Geometry check sheet. Reference: drawing and pictorial views, mm from the part's lowest x, y, z. A direction names the side the tool comes from. Coordinates: 2 decimals unless noted, no trailing zeros. Write each loop counter-clockwise with the first axis right and the second up, starting at its lowest first coordinate (ties: lowest second). Pieces come first, ordered by that corner, then holes. Notation, with made-up numbers: (34, 43.5) -> (45, 43.5) arc R23 ccw to (45, 67.5) -> close; hole circle Ø10 at (51.25, 38). An arc over 180 degrees is marked (long way). Answer in a Markdown table with one row per item.
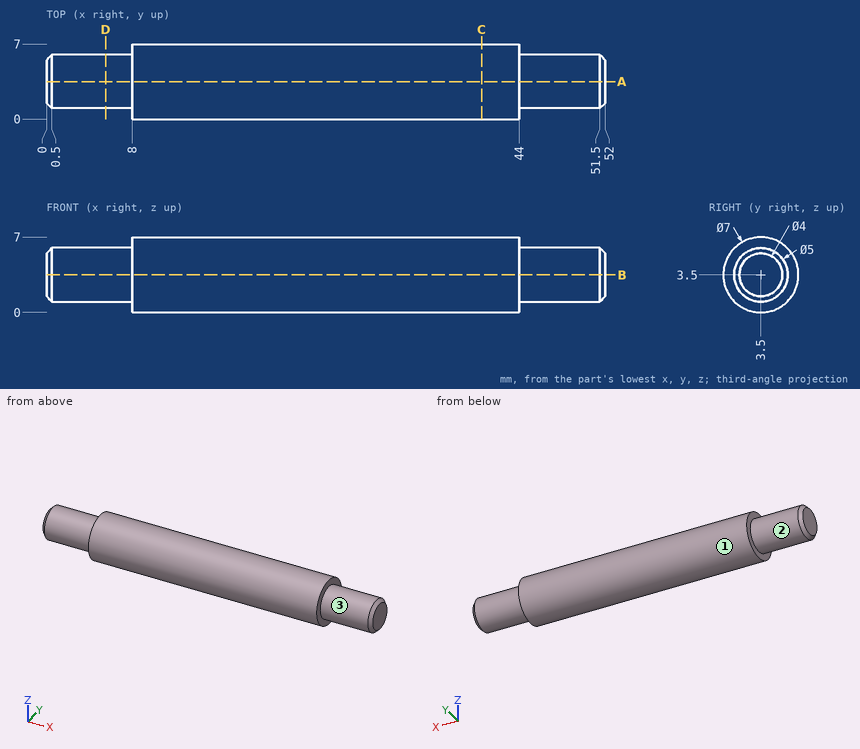
1. Section check A-A, the plane y = 3.5. Record the boundary of the cut face in (x, z).
Geometry says:
| item | result |
|---|---|
| outline | (0, 1.5) -> (0.5, 1) -> (8, 1) -> (8, 0) -> (44, 0) -> (44, 1) -> (51.5, 1) -> (52, 1.5) -> (52, 5.5) -> (51.5, 6) -> (44, 6) -> (44, 7) -> (8, 7) -> (8, 6) -> (0.5, 6) -> (0, 5.5) -> close |
2. Depth check by flat-ended pin: P1, Ø1.5, axis at x = 31, y = 5.5, coming from the +Z side; P2, Ø2, axis at x = 43, z = 1, coming from the +Y side; P3, Ø2, axis at x = 6, y = 6, coming from the +Z side. Enter the tip coordinate at first touch or a pass-through.
Geometry says:
| item | result |
|---|---|
| P1 | z = 6.77 |
| P2 | y = 6.66 |
| P3 | z = 5.5 |
3. Section check D-D, the plane x = 5.5. Record the boundary of the cut face in (y, z), plus the area to 3 significant figures.
Geometry says:
| item | result |
|---|---|
| outline | circle Ø5 at (3.5, 3.5) |
| area | 19.6 mm^2 |
4. Section check C-C, the plane x = 40.5. Record the boundary of the cut face in (y, z).
Geometry says:
| item | result |
|---|---|
| outline | circle Ø7 at (3.5, 3.5) |
5. Tool access check on the marked faces 1, 2 and 3. Record the directions out of +Z, -Z, +X, -X, +Y, -Y that give a thin tool (end or side, any length) a straight path to the whole face; none if there is none.
Geometry says:
| item | result |
|---|---|
| face 1 | +X, -X |
| face 2 | -X |
| face 3 | +X |
6. Thickness scan on line 1 (X direction, y = 6.25, z = 2); line 2 (Y direction, x = 6.5, z = 5.5); line 3 (Z direction, x = 41, y = 5.75). Record the ranges inside material, lowest first. Write a range as from..to.
Geometry says:
| item | result |
|---|---|
| line 1 | 8..44 |
| line 2 | 2..5 |
| line 3 | 0.82..6.18 |
